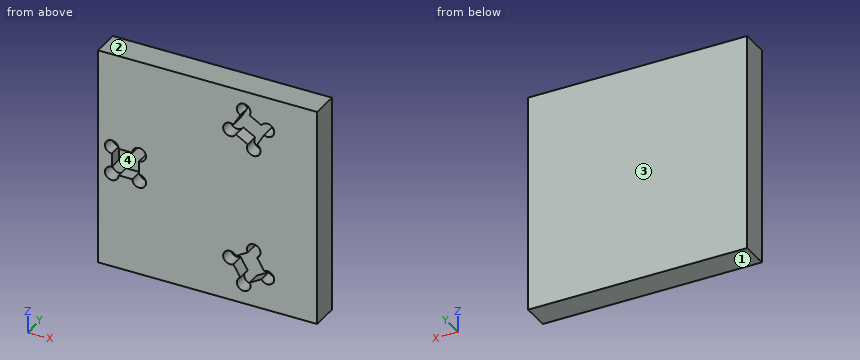
from build123d import *

# Parameters (mm, degrees)
SKETCH1_W           = 25.4
SKETCH1_H           = 25.4
BOSS_EXTRUDE1_DEPTH = 3.175
SKETCH2_R           = 0.79375
SKETCH2_W           = 3.175
SKETCH2_H           = 3.175
CUT_EXTRUDE1_DEPTH  = 1.5875


with BuildPart() as part:
    # Sketch1 → Boss-Extrude1 (new body)
    with BuildSketch(Plane(origin=(0, 0, 0), x_dir=(1, 0, 0), z_dir=(0, 1, 0))):
        Rectangle(SKETCH1_W, SKETCH1_H)
    extrude(amount=BOSS_EXTRUDE1_DEPTH)

    # Sketch2 → Cut-Extrude1 (cut)
    with BuildSketch(Plane.XZ):
        with Locations((-11.1125, -1.5875)):
            Circle(SKETCH2_R)
        with Locations((-11.1125, 1.5875)):
            Circle(SKETCH2_R)
        with Locations((-7.9375, 1.5875)):
            Circle(SKETCH2_R)
        with Locations((-7.9375, -1.5875)):
            Circle(SKETCH2_R)
        with Locations((4.181434671, 10.4174573)):
            Circle(SKETCH2_R)
        with Locations((6.931065329, 8.8299573)):
            Circle(SKETCH2_R)
        with Locations((5.343565329, 6.080326643)):
            Circle(SKETCH2_R)
        with Locations((2.593934671, 7.667826643)):
            Circle(SKETCH2_R)
        with Locations((6.931065329, -8.8299573)):
            Circle(SKETCH2_R)
        with Locations((4.181434671, -10.4174573)):
            Circle(SKETCH2_R)
        with Locations((2.593934671, -7.667826643)):
            Circle(SKETCH2_R)
        with Locations((5.343565329, -6.080326643)):
            Circle(SKETCH2_R)
        with Locations((-9.525, 0)):
            Rectangle(SKETCH2_W, SKETCH2_H)
        Polygon((6.931065329, 8.8299573), (4.181434671, 10.4174573), (2.593934671, 7.667826643), (5.343565329, 6.080326643), align=None)
        Polygon((4.181434671, -10.4174573), (6.931065329, -8.8299573), (5.343565329, -6.080326643), (2.593934671, -7.667826643), align=None)
    extrude(amount=-CUT_EXTRUDE1_DEPTH, mode=Mode.SUBTRACT)


solid = part.part
Can you work these out from the model? Positions are in its coordinate system, mm. Face numbers are marked on the shaded views. Give positions to 0.01 mm unless a question says otherwise; leave off trailing zeros. Order: outer loops, then holes, each group sorted by start corner. A loop starts at its lowest first (then second) coordinate and runs counter-clockwise, first axis right, second up. Notation, with made-up numbers: M 4.5,27 L 47.5,27 A23 ccw 47.5,38 Z; hole C 46.25,11 d3. An arc over 180 degrees is marked long. Use a Markdown table: item, result. Add a question column.
Item 1: Suppose I cut it at B-B (x = -9.25). List the corners of the cut face in (y, z) for me (1 decimal), then the cut area to 3 significant figures.
Item 2: Will this pin go through, and if not, where does the flat tip stop? pin 1 (1.4 mm diameter, centred on x = 2.59, z = 7.67, fed in from -Y).
Item 3: If I drill on L1, parallel to Z at x = 2.5, y = 1.55; L2, parallel to Z at x = 2, y = 1.45; L3, parallel to Y at x = -10.5, z = 0 (1 decimal), over which ranges is the centre line in solid material (lowest first)? Write a range as [from, to].
Item 4: Suppose I cut it at A-A (y = 1.05). List the corners of the cut face in (x, z) for me.
Item 5: We'd pull the mould along Z, two halves only. Please class the marked faces 1, 2, 3 and 4: +Z half, -Z half, draft (parallel to the pull), parting line (faces both ways), or undercut.
Answer sheet:
| question | item | result |
|---|---|---|
| 1 | outline | M 0,-12.7 L 3.2,-12.7 L 3.2,12.7 L 0,12.7 L 0,1.6 L 1.6,1.6 L 1.6,-1.6 L 0,-1.6 Z |
| 1 | area | 75.6 mm² |
| 2 | pin 1 | stops at y = 1.59 |
| 3 | L1 | z = [-12.7, -8.46], [-6.88, 6.88], [8.46, 12.7] |
| 3 | L2 | z = [-12.7, -8.19], [-7.14, 7.14], [8.19, 12.7] |
| 3 | L3 | y = [1.6, 3.2] |
| 4 | outline | M -12.7,-12.7 L 12.7,-12.7 L 12.7,12.7 L -12.7,12.7 Z; hole M -11.11,-0.79 A0.79 ccw long -10.32,-1.59 L -8.73,-1.59 A0.79 ccw long -7.94,-0.79 L -7.94,0.79 A0.79 ccw long -8.73,1.59 L -10.32,1.59 A0.79 ccw long -11.11,0.79 Z; hole M 2.99,-8.36 L 3.78,-9.73 A0.79 ccw long 4.87,-10.02 L 6.24,-9.23 A0.79 ccw long 6.53,-8.14 L 5.74,-6.77 A0.79 ccw long 4.66,-6.48 L 3.28,-7.27 A0.79 ccw long Z; hole M 2.99,8.36 A0.79 ccw long 3.28,7.27 L 4.66,6.48 A0.79 ccw long 5.74,6.77 L 6.53,8.14 A0.79 ccw long 6.24,9.23 L 4.87,10.02 A0.79 ccw long 3.78,9.73 Z |
| 5 | face 1 | -Z half |
| 5 | face 2 | +Z half |
| 5 | face 3 | draft |
| 5 | face 4 | undercut |
